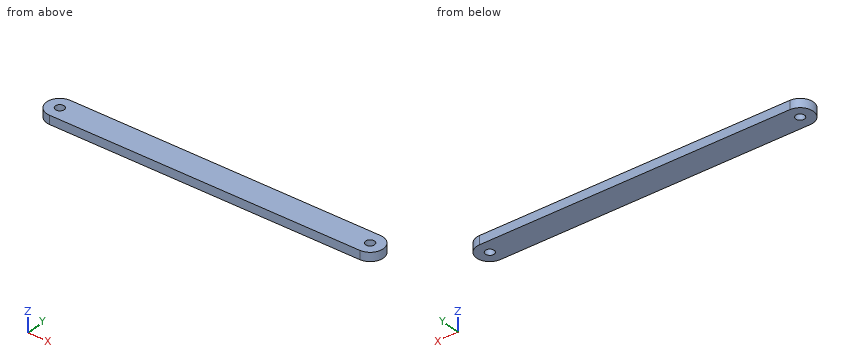
Autodesk Inventor part; units mm, degrees
ref_plane "YZ Plane" through (0, 0, 0) normal (1, 0, 0) x (0, 1, 0)
ref_plane "XZ Plane" through (0, 0, 0) normal (0, 1, 0) x (-1, 0, 0)
ref_plane "XY Plane" through (0, 0, 0) normal (0, 0, 1) x (1, 0, 0)
sketch "Sketch1" plane through (0, 0, 0) normal (0, 0, 1) x (1, 0, 0)
  circle A0 centre (-35, 0) radius 1
  circle A1 centre (35, 0) radius 1
  line L0 (-35, 0) -> (0, 0) construction
  line L1 (0, 0) -> (35, 0) construction
  line L2 (-35, 3) -> (35, 3)
  line L3 (-35, -3) -> (35, -3)
  line L4 (0, 3) -> (0, -3) construction
  arc A2 (-35, 3) -> (-35, -3) centre (-35, 0) ccw
  arc A3 (35, -3) -> (35, 3) centre (35, 0) ccw
  point P0 (-35, -1)
  dimension "d0" = 2
  dimension "d1" = 2
  dimension "d2" = 35
extrude "Extrusion1" add sketch "Sketch1" along normal blind 2
properties part number "LongLink"
For this review, take the finished solid that the model builds, in its own axes (mm). Round coordinates to 2 decimals unless told otherwise and drop trailing zeros. Write each loop counter-clockwise with the first axis right and the second up, starting at its lowest first coordinate (ties: lowest second). Pieces come first, ordered by that corner, then holes. Notation, with made-up numbers: (51, 67) - (59, 67) arc R18 cw to (59, 100) - close; hole circle Ø7 at (17.5, 49). An arc over 180 degrees is marked (long way). Use a Markdown table: item, result.
Q1. We need section A-A (z = 1.2). Give the boundary of the cut face in (x, y).
Derived:
| item | result |
|---|---|
| outline | (-35, -3) - (35, -3) arc R3 ccw to (35, 3) - (-35, 3) arc R3 ccw to start; hole circle Ø2 at (-35, 0); hole circle Ø2 at (35, 0) |
Q2. Clearance check with a flat-ended pin moving along its axis: pin 1 (2.5 mm diameter, centred on x = -35, y = 0, fed in from +Z). State where the tip first meets the part, or that it passes through.
Derived:
| item | result |
|---|---|
| pin 1 | stops at z = 2 |
Q3. We need section B-B (y = 0). Give the boundary of the cut face in (x, z).
Derived:
| item | result |
|---|---|
| outline | (-38, 0) - (-36, 0) - (-36, 2) - (-38, 2) - close; (-34, 0) - (34, 0) - (34, 2) - (-34, 2) - close; (36, 0) - (38, 0) - (38, 2) - (36, 2) - close |
Q4. Wall thickness on line 1 along X through (y, z) = (-0.3, 1.05); line 2 along Y through (x, z) = (-35, 1.45); line 3 along X through (y, z) = (2.1, 1.05): over which ranges is each line inside the solid? List them lowest first.
Derived:
| item | result |
|---|---|
| line 1 | x = -37.98 to -35.95, -34.05 to 34.05, 35.95 to 37.98 |
| line 2 | y = -3 to -1, 1 to 3 |
| line 3 | x = -37.14 to 37.14 |
